Solid Edge part; units mm, degrees
sketch "Sketch1" plane through (0, 0, 0) normal (0, 0, 1) x (1, 0, 0)
  line L0 (-31.6, -7.05) -> (31.6, -7.05)
  line L1 (31.6, -7.05) -> (31.6, 7.05)
  line L2 (31.6, 7.05) -> (-31.6, 7.05)
  line L3 (-31.6, 7.05) -> (-31.6, -7.05)
  circle A0 centre (-24.55, 0) radius 2.05
  circle A1 centre (-15.4, 0) radius 2.1
  circle A2 centre (-6.15, 0) radius 2.15
  circle A3 centre (3.55, 0) radius 2.55
  circle A4 centre (13.7, 0) radius 2.6
  circle A5 centre (23.95, 0) radius 2.65
extrude "Protrusion1" add sketch "Sketch1" along normal blind 10
For this review, take the finished solid that the model builds, in its own axes (mm). Give positions to 0.01 mm unless a question says otherwise; leave off trailing zeros. Order: outer loops, then holes, each group sorted by start corner. A loop starts at its lowest first (then second) coordinate and runs counter-clockwise, first axis right, second up.
1) The part is to be moulded in two halves that separate along Y. For faces 1 (the face through (-8.3, -0.09, 4.93)), 2 (the face through (0, -7.05, 5)), 3 (the face through (31.6, 0, 5)), say which applies: released by +Y, released by -Y, zero draft, split by the parting line, or undercut.
2) Take a section at A-A (x = -15.4). Give the boundary of the cut face in (y, z), then the cut area to 3 significant figures.
3) Take a section at D-D (x = 3.55). Give the boundary of the cut face in (y, z).
4) Take a section at B-B (z = 1). Give the boundary of the cut face in (x, y).
5) Take a section at C-C (y = -1.25). Give the boundary of the cut face in (x, z), then the cut area to 3 significant figures.
6) Wall thickness on line 1 (Y direction, x = -6.15, z = 3.25); line 2 (Y direction, x = -24.55, z = 6); line 3 (X direction, y = 2.25, z = 4): over which ranges is each line inside the solid? List them lowest first.
7) Insertion check: pin 1 (3 mm diameter, centred on x = 13.7, y = 0, fed in from -Z). The pin has a flat end and moves straight along its axis. Give the tip position at first contact, or say it passes through.
Derived:
1. face 1: undercut
1. face 2: released by -Y
1. face 3: zero draft
2. outline: (-7.05, 0) - (-2.1, 0) - (-2.1, 10) - (-7.05, 10) - close; (2.1, 0) - (7.05, 0) - (7.05, 10) - (2.1, 10) - close
2. area: 99.0 mm2
3. outline: (-7.05, 0) - (-2.55, 0) - (-2.55, 10) - (-7.05, 10) - close; (2.55, 0) - (7.05, 0) - (7.05, 10) - (2.55, 10) - close
4. outline: (-31.6, -7.05) - (31.6, -7.05) - (31.6, 7.05) - (-31.6, 7.05) - close; hole circle Ø4.1 at (-24.55, 0); hole circle Ø4.2 at (-15.4, 0); hole circle Ø4.3 at (-6.15, 0); hole circle Ø5.1 at (3.55, 0); hole circle Ø5.2 at (13.7, 0); hole circle Ø5.3 at (23.95, 0)
5. outline: (-31.6, 0) - (-26.17, 0) - (-26.17, 10) - (-31.6, 10) - close; (-22.93, 0) - (-17.09, 0) - (-17.09, 10) - (-22.93, 10) - close; (-13.71, 0) - (-7.9, 0) - (-7.9, 10) - (-13.71, 10) - close; (-4.4, 0) - (1.33, 0) - (1.33, 10) - (-4.4, 10) - close; (5.77, 0) - (11.42, 0) - (11.42, 10) - (5.77, 10) - close; (15.98, 0) - (21.61, 0) - (21.61, 10) - (15.98, 10) - close; (26.29, 0) - (31.6, 0) - (31.6, 10) - (26.29, 10) - close
5. area: 394 mm2
6. line 1: y = -7.05 to -2.15, 2.15 to 7.05
6. line 2: y = -7.05 to -2.05, 2.05 to 7.05
6. line 3: x = -31.6 to 2.35, 4.75 to 12.4, 15 to 22.55, 25.35 to 31.6
7. pin 1: passes through
